Model file for the job. Use its own axes, mm. Face numbers are marked on the shaded views. Round coordinates to 2 decimals unless told otherwise and drop trailing zeros. Order: outer loops, then holes, each group sorted by start corner. A loop starts at its lowest first (then second) coordinate and runs counter-clockwise, first axis right, second up. Notation, with made-up numbers: (21.5, 0.25) - (70.5, 0.25) arc R18 ccw to (70.5, 10.25) - close; hole circle Ø10 at (-34.75, 88.25). An arc over 180 degrees is marked (long way). Put each result on its own line as item: value. Start each with the question number.
Item 1: Saw through at B-B on x = 12.2. List the corners of the cut face in (y, z).
Item 2: Mould opens along Z. For the marked faces 1 and 2 say: pulls with the +Z half, pulls with the -Z half, needs draft (parallel to the pull), parting line crosses it, or undercut.
Item 3: Saw through at C-C on x = -8. List the corners of the cut face in (y, z).
Item 4: Saw through at D-D on z = 7. List the corners of the cut face in (x, y).
Item 5: Pin check, flat tips, straight feed: pin 1 Ø6.5 at (x, z) = (12.2, 0) entering from +Y; pin 2 Ø4 at (y, z) = (-5, 5) entering from +X; pin 3 Ø4 at (y, z) = (-5, -6.5) entering from +X; pin 4 Ø1.5 at (x, y) = (4, -8.5) entering from +Z. Stop position of each tip, or through.
Item 6: Saw through at A-A on y = -2.75. List the corners of the cut face in (x, z), plus the area to 3 significant figures.
Item 7: Probe probe 1 along Z at (x, y) = (12.2, -4.75); probe 2 along X at (y, z) = (-3.5, 0.25); probe 3 along X at (y, z) = (-4.25, -3.5). List the from-to ranges inside material, lowest first.
```python
from build123d import *

# Parameters (mm, degrees)
F0_R     = 4
F1_DEPTH = 10
F0_R_2   = 2
F2_DEPTH = 10
F3_DEPTH = 10


with BuildPart() as f1:
    # F0 (on Front) → F1 (new body)
    with BuildSketch(Plane.XZ):
        with BuildLine():
            ThreePointArc((9.7654713115, -2.1530374044), (8.95, 0), (9.7654713115, 2.1530374044))
            ThreePointArc((9.7654713115, 2.1530374044), (0, 10), (-9.7654713115, 2.1530374044))
            ThreePointArc((-9.7654713115, 2.1530374044), (-9.1606975934, 1.1511476366), (-8.95, 0))
            ThreePointArc((-8.95, 0), (-9.1606975934, -1.1511476366), (-9.7654713115, -2.1530374044))
            ThreePointArc((-9.7654713115, -2.1530374044), (0, -10), (9.7654713115, -2.1530374044))
        make_face()
        with Locations((-4.5, 0)):
            Circle(F0_R, mode=Mode.SUBTRACT)
        with Locations((4.5, 0)):
            Circle(F0_R, mode=Mode.SUBTRACT)
    extrude(amount=F1_DEPTH)

    # F0 (on Front) → F2 (join)
    with BuildSketch(Plane.XZ):
        with BuildLine():
            ThreePointArc((-9.7654713115, -2.1530374044), (-10, 0), (-9.7654713115, 2.1530374044))
            ThreePointArc((-9.7654713115, 2.1530374044), (-15.45, 0), (-9.7654713115, -2.1530374044))
        make_face()
        with Locations((-12.2, 0)):
            Circle(F0_R_2, mode=Mode.SUBTRACT)
        with BuildLine():
            ThreePointArc((9.7654713115, 2.1530374044), (9.941194926, 1.082886625), (10, 0))
            ThreePointArc((10, 0), (9.941194926, -1.082886625), (9.7654713115, -2.1530374044))
            ThreePointArc((9.7654713115, -2.1530374044), (13.3511476366, -3.0393024066), (15.45, 0))
            ThreePointArc((15.45, 0), (13.3511476366, 3.0393024066), (9.7654713115, 2.1530374044))
        make_face()
        with Locations((12.2, 0)):
            Circle(F0_R_2, mode=Mode.SUBTRACT)
    extrude(amount=F2_DEPTH)

    # F0 (on Front) → F3 (join)
    with BuildSketch(Plane.XZ):
        with BuildLine():
            ThreePointArc((9.7654713115, -2.1530374044), (9.941194926, -1.082886625), (10, 0))
            ThreePointArc((10, 0), (9.941194926, 1.082886625), (9.7654713115, 2.1530374044))
            ThreePointArc((9.7654713115, 2.1530374044), (8.95, 0), (9.7654713115, -2.1530374044))
        make_face()
        with BuildLine():
            ThreePointArc((-8.95, 0), (-9.1606975934, 1.1511476366), (-9.7654713115, 2.1530374044))
            ThreePointArc((-9.7654713115, 2.1530374044), (-10, 0), (-9.7654713115, -2.1530374044))
            ThreePointArc((-9.7654713115, -2.1530374044), (-9.1606975934, -1.1511476366), (-8.95, 0))
        make_face()
    extrude(amount=F3_DEPTH)


solid = f1.part
```
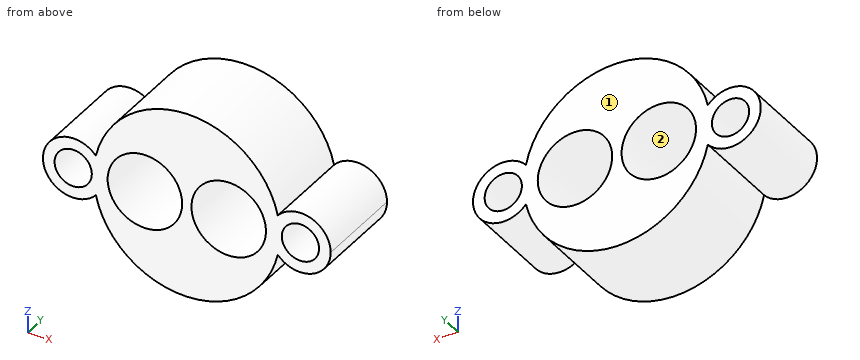
Results found:
1. outline: (-10, -3.25) - (0, -3.25) - (0, -2) - (-10, -2) - close; (-10, 2) - (0, 2) - (0, 3.25) - (-10, 3.25) - close
2. face 1: needs draft
2. face 2: undercut
3. outline: (-10, -6) - (0, -6) - (0, -1.94) - (-10, -1.94) - close; (-10, 1.94) - (0, 1.94) - (0, 6) - (-10, 6) - close
4. outline: (-7.14, -10) - (7.14, -10) - (7.14, 0) - (-7.14, 0) - close
5. pin 1: stops at y = 0
5. pin 2: stops at x = 13.45
5. pin 3: stops at x = 8.93
5. pin 4: stops at z = 9.46
6. outline: (-9.77, -2.15) arc R10 ccw to (9.77, -2.15) arc R3.25 ccw (long way) to (9.77, 2.15) arc R10 ccw to (-9.77, 2.15) arc R3.25 ccw (long way) to start; hole circle Ø4 at (-12.2, 0); hole circle Ø8 at (-4.5, 0); hole circle Ø8 at (4.5, 0); hole circle Ø4 at (12.2, 0)
6. area: 249 mm²
7. probe 1: z = -3.25 to -2, 2 to 3.25
7. probe 2: x = -15.44 to -14.18, -10.22 to -8.49, -0.51 to 0.51, 8.49 to 10.22, 14.18 to 15.44
7. probe 3: x = -9.37 to -6.44, -2.56 to 2.56, 6.44 to 9.37
